Can you work these out from the model? Positions are in its coordinate system, mm. A direction names the side the tool comes from. Coordinates: 2 decimals unless noted, no trailing zeros. Write each loop counter-clockwise with the first axis right and the second up, starting at its lowest first coordinate (ties: lowest second). Pieces come first, ordered by that corner, then holes. Notation, with made-up numbers: (32.25, -20) - (38.25, -20) arc R7 cw to (38.25, -11) - close; hole circle Ø2 at (89.25, 5.5). An arc over 180 degrees is marked (long way). Use one line per item in the form item = value. Start each with the question number.
(1) If I drill on probe 1 along X at (y, z) = (0, 1.15); probe 2 along Y at (x, z) = (6.5, 0.25); probe 3 along Z at (x, y) = (2.5, 5), over which ranges is the centre line in solid material (lowest first)? Write a range as from..to.
(2) If we section it at B-B on x = 6.5: Please give me the cut outline in (y, z), then the cut area to 3 significant figures.
(3) If we section it at D-D on z = -1: Please give me the cut outline in (x, y).
(4) If we section it at A-A on y = 0: Please give me the cut outline in (x, z), then the cut area to 4 significant figures.
(5) Thinking about a two-plate mould opening in X: for faces 1 (the face through (5, -1, -2)), 2 (the face through (1.5, 0, 6)), 3 (the face through (5, 0, 1)), which applies, pulls with the +X half, pulls with the -X half, needs draft (parallel to the pull), parting line crosses it, or undercut?
(6) For pin 1 Ø1.2 at (y, z) = (6, 4.5) entering from +X; pin 2 Ø1.5 at (y, z) = (-8, 2) entering from +X; pin 3 Ø1.5 at (y, z) = (10, -0.5) entering from +X, each with a flat end and sliding along its axis, tell me the tip position at first contact or that it passes through.
(7) On a 3-axis mill with a long thin cutter (end or side, diameter ignored), from which of +Z, -Z, +X, -X, +Y, -Y can I reach the whole of each face in a straight line? I mean faces 4 (the face through (9, -15, 2)), 5 (the face through (12.494, 0.264, -0.986)), 6 (the face through (2, 0, 7)), 7 (the face through (1, 0, 5.5)), 8 (the face through (14, 0, 3)). Say none if no direction works.
(8) If we section it at C-C on y = 7: Please give me the cut outline in (x, z).
```python
from build123d import *

# Parameters (mm, degrees)
EXTRU_MINCE1_DEPTH      = 15
ESQUISSE2_R             = 1.5
ENL_V_MAT_EXTRU_1_DEPTH = 32.144823005
ESQUISSE3_W             = 1.5
ESQUISSE3_H             = 1.5
ENL_V_MAT_EXTRU_2_DEPTH = 40.990623901
ESQUISSE4_R             = 6
ESQUISSE4_R_2           = 1.5
BOSS_EXTRU_1_DEPTH      = 2


with BuildPart() as part:
    # Esquisse1 → Extru.-Mince1 (new, symmetric)
    with BuildSketch(Plane(origin=(0, 0, 0), x_dir=(1, 0, 0), z_dir=(0, 1, 0))):
        Polygon((0, -7), (0, 0), (27, 0), (27, -3), (3, -3), (3, -7), align=None)
    extrude(amount=EXTRU_MINCE1_DEPTH, both=True)

    # Esquisse2 → Enlèv. mat.-Extru.1 (cut, through all)
    with BuildSketch(Plane.XY.offset(3)):
        with Locations((6.5, 0)):
            Circle(ESQUISSE2_R)
        with BuildLine():
            Line((18.16190379, -15), (27, -15))
            Line((27, -15), (27, 15))
            Line((27, 15), (18.16190379, 15))
            ThreePointArc((18.16190379, 15), (25.5, 0), (18.16190379, -15))
        make_face()
    extrude(amount=-ENL_V_MAT_EXTRU_1_DEPTH, mode=Mode.SUBTRACT)

    # Esquisse3 → Enlèv. mat.-Extru.2 (cut, through all)
    with BuildSketch(Plane(origin=(0, 15, 0), x_dir=(1, 0, 0), z_dir=(0, 1, 0))):
        with Locations((0.75, -6.25)):
            Rectangle(ESQUISSE3_W, ESQUISSE3_H)
    extrude(amount=-ENL_V_MAT_EXTRU_2_DEPTH, mode=Mode.SUBTRACT)

    # Esquisse4 → Boss.-Extru.1 (add)
    with BuildSketch(Plane(origin=(0, 0, 0), x_dir=(-1, 0, 0), z_dir=(0, 0, -1))):
        with Locations((-6.5, 0)):
            Circle(ESQUISSE4_R)
        with Locations(Location((-6.5, 0, 0), (0, 0, 180))):
            Circle(ESQUISSE4_R_2, mode=Mode.SUBTRACT)
    extrude(amount=BOSS_EXTRU_1_DEPTH)


solid = part.part
```
Reported:
q1.probe_1 = 0..5, 8..25.5
q1.probe_2 = -15..-1.5, 1.5..15
q1.probe_3 = 0..7
q2.outline = (-15, 0) - (-6, 0) - (-6, -2) - (-1.5, -2) - (-1.5, 3) - (-15, 3) - close; (1.5, -2) - (6, -2) - (6, 0) - (15, 0) - (15, 3) - (1.5, 3) - close
q2.area = 99.0 mm2
q3.outline = circle Ø12 at (6.5, 0); hole circle Ø3 at (6.5, 0)
q4.outline = (0, 0) - (0.5, 0) - (0.5, -2) - (5, -2) - (5, 3) - (3, 3) - (3, 7) - (1.5, 7) - (1.5, 5.5) - (0, 5.5) - close; (8, -2) - (12.5, -2) - (12.5, 0) - (25.5, 0) - (25.5, 3) - (8, 3) - close
q4.area = 95.25 mm2
q5.face_1 = needs draft
q5.face_2 = pulls with the -X half
q5.face_3 = undercut
q6.pin_1 = 3
q6.pin_2 = 24.06
q6.pin_3 = 22.99
q7.face_4 = +Z, -Z, +X, -X, -Y
q7.face_5 = -Z
q7.face_6 = +Z, +X, -X, +Y, -Y
q7.face_7 = +Z, -X, +Y, -Y
q7.face_8 = +Z, +X, +Y, -Y
q8.outline = (0, 0) - (24.16, 0) - (24.16, 3) - (3, 3) - (3, 7) - (1.5, 7) - (1.5, 5.5) - (0, 5.5) - close
